```python
from build123d import *

# Parameters (mm, degrees)
ESQUISSE1_R        = 1.75
BOSS_EXTRU_1_DEPTH = 2
CONG_1_R           = 3.5


with BuildPart() as part:
    # Esquisse1 → Boss.-Extru.1 (new body)
    with BuildSketch(Plane.XY):
        Polygon((-64.5, 9), (-29.5, 9), (-29.5, -12.5), (26, -12.5), (26, -21.5), (33, -21.5), (33, -12.5), (33, 16), (-29.5, 16), (-64.5, 16), align=None)
        with Locations((29.5, -17.5)):
            Circle(ESQUISSE1_R, mode=Mode.SUBTRACT)
        with Locations((-60.5, 12.5)):
            Circle(ESQUISSE1_R, mode=Mode.SUBTRACT)
    extrude(amount=BOSS_EXTRU_1_DEPTH)

    # Congé1
    cong_1_edges = [part.edges().sort_by_distance(p)[0] for p in [
        (33, 16, 1),
        (26, -12.5, 1),
        (-29.5, -12.5, 1),
        (-29.5, 9, 1),
        (-64.5, 16, 1),
        (-64.5, 9, 1),
        (26, -21.5, 1),
        (33, -21.5, 1),
    ]]
    fillet(cong_1_edges, radius=CONG_1_R - 0.0001)  # a hair under: the kernel refuses the full size


solid = part.part
```
Model file for the job. Use its own axes, mm. A direction names the side the tool comes from. Give positions to 0.01 mm unless a question says otherwise; leave off trailing zeros. Write each loop counter-clockwise with the first axis right and the second up, starting at its lowest first coordinate (ties: lowest second). Pieces come first, ordered by that corner, then holes. Notation, with made-up numbers: (12, 87.25) - (53, 87.25) arc R9 ccw to (53, 104.25) - close; hole circle Ø6 at (81.5, 28). An arc over 180 degrees is marked (long way). One line per question, with ' | ' between items. Start each with the question number.
(1) 3-axis set-ups, long thin cutter, end or side, ignore diameter. For faces 1 (the face through (-2, -12.5, 1)), 2 (the face through (-6, 2, 2)): which of +Z, -Z, +X, -X, +Y, -Y reach the whole face in a straight line?
(2) Slice it at C-C on y = -6. Write the cut outline in (x, z).
(3) Two-plate mould, pull along Y, no slides. Class faces 3 (the face through (-58.831, 13.026, 0.986)), 4 (the face through (33, -3, 1)), 5 (the face through (32, -20.45, 1.01)), 6 (the face through (-63.5, 14.95, 1.01)): +Y half, -Y half, draft (parallel to the pull), parting line (faces both ways), or undercut.
(4) Pin check, flat tip, straight feed: P1, Ø1, axis at y = 0, z = 1.5, coming from the -X side. Stop position of the tip, or through.
(5) Wall check: line 1 along Y through (x, z) = (29.5, 0.5); line 2 along Y through (x, z) = (-10, 1.9); line 3 along X through (y, z) = (-3.5, 0.65). Give the ranges that are in metal, low to high. Write a range as from..to.
(6) Slice it at B-B on x = -46.5. Write the cut outline in (y, z).
(7) Slice it at A-A on z = 0.5. Give the number of separate pieces and of enclosed holes in the cut face, plus the area to 3 significant figures.
Results below:
1) face 1: +Z, -Z, -X, -Y | face 2: +Z, +X, -X, +Y, -Y
2) outline: (-29.5, 0) - (33, 0) - (33, 2) - (-29.5, 2) - close
3) face 3: undercut | face 4: draft | face 5: -Y half | face 6: +Y half
4) P1: x = -29.5
5) line 1: -21.5..-19.25, -15.75..16 | line 2: -12.5..16 | line 3: -29.5..33
6) outline: (9, 0) - (16, 0) - (16, 2) - (9, 2) - close
7) separate pieces: 1 | enclosed holes: 2 | area: 2,060 mm^2
